Read the model definition and answer for the solid it produces. Units are mm, in the model's axes. Coordinates: 2 decimals unless noted, no trailing zeros. Loops run counter-clockwise (first coordinate to the right, second up) from the corner with the lowest first, then second, coordinate; pieces in that order, holes last.
from build123d import *

# Parameters (mm, degrees)
SKETCH1_R           = 2.032
BOSS_EXTRUDE1_DEPTH = 3.175


with BuildPart() as part:
    # Sketch1 → Boss-Extrude1 (new body)
    with BuildSketch(Plane.XY):
        with BuildLine():
            Line((-6.300195309, -26.19375), (-9.450292964, -1.190625))
            ThreePointArc((-9.450292964, -1.190625), (-6.434996728, 7.022566633), (2.009741615, 9.31056194))
            Line((2.009741615, 9.31056194), (26.643173075, 3.993285428))
            ThreePointArc((26.643173075, 3.993285428), (31.376812055, -4.067266578), (22.949101168, -8.111215863))
            ThreePointArc((22.949101168, -8.111215863), (9.660617203, -10.542713679), (6.08020428, -23.568711952))
            ThreePointArc((6.08020428, -23.568711952), (1.317120041, -31.611899452), (-6.300195309, -26.19375))
        make_face()
        Circle(SKETCH1_R, mode=Mode.SUBTRACT)
        with Locations((25.303345332, -2.213755866)):
            Circle(SKETCH1_R, mode=Mode.SUBTRACT)
        with Locations((0, -25.4)):
            Circle(SKETCH1_R, mode=Mode.SUBTRACT)
    extrude(amount=BOSS_EXTRUDE1_DEPTH)


solid = part.part
Q1. A cutting plane is placed at D-D (y = -16). Give the vertices of the cut face in (x, z) (3 decimals).
Findings below:
outline: (-7.584, 0) - (6.156, 0) - (6.156, 3.175) - (-7.584, 3.175) - close
Q2. Flat-ended cylindrical pins translate along their axes: pin 1 Ø6.5 at (x, y) = (0, -25.4) entering from -Z; pin 2 Ø1 at (y, z) = (-19.5, 0.5) entering from -X; pin 3 Ø1.5 at (y, z) = (-12.5, 1) entering from -X; pin 4 Ø1 at (x, z) = (-3, 2.5) entering from +Y. Find the tip coordinate at first contact, or state that the pin passes through.
Findings below:
pin 1: stops at z = 0
pin 2: stops at x = -7.21
pin 3: stops at x = -8.12
pin 4: stops at y = 9.19
Q3. A cutting plane is placed at C-C (z = 1.8). Give the vertices of the cut face in (x, y) (3 decimals).
Findings below:
outline: (-9.45, -1.191) - (-6.3, -26.194) arc R6.35 ccw (long way) to (6.08, -23.569) arc R12.7 cw to (22.949, -8.111) arc R6.35 ccw (long way) to (26.643, 3.993) - (2.01, 9.311) arc R9.525 ccw to start; hole circle Ø4.064 at (0, -25.4); hole circle Ø4.064 at (0, 0); hole circle Ø4.064 at (25.303, -2.214)
Q4. A cutting plane is placed at A-A (x = 0). Give the vertices of the cut face in (y, z) (3 decimals).
Findings below:
outline: (-31.75, 0) - (-27.432, 0) - (-27.432, 3.175) - (-31.75, 3.175) - close; (-23.368, 0) - (-2.032, 0) - (-2.032, 3.175) - (-23.368, 3.175) - close; (2.032, 0) - (9.525, 0) - (9.525, 3.175) - (2.032, 3.175) - close
Q5. Determine the mould class of faces 1 (the face through (14.15, 6.69, 1.57)), 2 (the face through (-7.853, -13.867, 1.565)), 3 (the face through (-0.44, -27.384, 1.565)), 4 (the face through (-0.44, -1.984, 1.565)) for opening direction X: +X half, -X half, draft (parallel to the pull), parting line (faces both ways), or undercut.
Findings below:
face 1: +X half
face 2: -X half
face 3: undercut
face 4: undercut
Q6. A cutting plane is placed at B-B (y = -25.4). Give the vertices of the cut face in (x, z) (3 decimals), then the cut area to 3 significant figures.
Findings below:
outline: (-6.4, 0) - (-2.032, 0) - (-2.032, 3.175) - (-6.4, 3.175) - close; (2.032, 0) - (6.35, 0) - (6.35, 3.175) - (2.032, 3.175) - close
area: 27.6 mm2
Q7. Straight lines are drawn through the part: probe 1 along Y at (x, z) = (0, 0.85) (3 decimals); probe 2 along X at (y, z) = (-2.5, 1.75); probe 3 along Y at (x, z) = (13.5, 2.75). For each, find the intervals that lie inside material, in ascending order.
Findings below:
probe 1: y = -31.75 to -27.432, -23.368 to -2.032, 2.032 to 9.525
probe 2: x = -9.29 to 23.29, 27.32 to 31.65
probe 3: y = -8.12 to 6.83
